Input: part model. Units: mm. Frame: model coordinates. Round coordinates to 2 decimals unless told otherwise and drop trailing zeros. Order: outer loops, then holes, each group sorted by start corner. A loop starts at its lowest first (then second) coordinate and runs counter-clockwise, first axis right, second up. Notation, with made-up numbers: (71.5, 49.25) -> (123.5, 49.25) arc R18 cw to (123.5, 57.25) -> close; hole circle Ø7 at (39, -1). An arc over 180 degrees is marked (long way). Use a Markdown table: item, result.
Autodesk Inventor part; units mm, degrees
ref_plane "YZ Plane" through (0, 0, 0) normal (1, 0, 0) x (0, 1, 0)
ref_plane "XZ Plane" through (0, 0, 0) normal (0, 1, 0) x (-1, 0, 0)
ref_plane "XY Plane" through (0, 0, 0) normal (0, 0, 1) x (1, 0, 0)
sketch "Sketch1" plane through (0, 0, 0) normal (0, 0, 1) x (1, 0, 0)
  line L0 (0, 0) -> (200, 0)
  line L1 (200, 0) -> (200, 200)
  line L2 (200, 200) -> (0, 200)
  line L3 (0, 200) -> (0, 0)
  circle A0 centre (10, 190) radius 3
  circle A1 centre (190, 190) radius 3
  circle A2 centre (190, 10) radius 3
  circle A3 centre (10, 10) radius 3
  circle A4 centre (61.1091, 138.8909) radius 3
  circle A5 centre (61.1091, 61.1091) radius 3
  circle A6 centre (138.8909, 61.1091) radius 3
  circle A7 centre (138.8909, 138.8909) radius 3
  point P0 (164, 100)
  dimension "d1" = 200
  dimension "d5" = 10
  dimension "d6" = 10
  dimension "d7" = 10
  dimension "d8" = 10
  dimension "d9" = 6
  dimension "d10" = 6
  dimension "d11" = 10
  dimension "d12" = 10
  dimension "d14" = 10
  dimension "d15" = 6
  dimension "d16" = 6
  dimension "d17" = 6
  dimension "d18" = 6
  dimension "d19" = 6
  dimension "d20" = 6
  dimension "d42" = 200
  dimension "d43" = 10
extrude "Extrusion2" add sketch "Sketch1" along normal blind 10
thread "Thread1"
thread "Thread2"
thread "Thread3"
thread "Thread4"
properties part number "PhlangeForShop"
1) Draft query along X for faces 1 (the face through (10, 187, 5)), 2 (the face through (99, 101, 10)), 3 (the face through (200, 99, 5)). Return one class per face: released by +X, released by -X, zero draft, split by the parting line, or undercut.
Answer key:
| item | result |
|---|---|
| face 1 | undercut |
| face 2 | zero draft |
| face 3 | released by +X |
2) Cut plane A-A on x = 190. Return loops of the section in (y, z).
Answer key:
| item | result |
|---|---|
| outline | (0, 0) -> (7, 0) -> (7, 10) -> (0, 10) -> close; (13, 0) -> (187, 0) -> (187, 10) -> (13, 10) -> close; (193, 0) -> (200, 0) -> (200, 10) -> (193, 10) -> close |
3) Ray query, probe 1 along X at (y, z) = (190, 5); probe 2 along X at (y, z) = (9, 6.5). Return the intervals inside material, ascending.
Answer key:
| item | result |
|---|---|
| probe 1 | x = 0 to 7, 13 to 187, 193 to 200 |
| probe 2 | x = 0 to 7.17, 12.83 to 187.17, 192.83 to 200 |
